from build123d import *

# Parameters (mm, degrees)
SKETCH1_R           = 40
BOSS_EXTRUDE1_DEPTH = 100
SKETCH2_R           = 30
SKETCH2_R_2         = 15
BOSS_EXTRUDE2_DEPTH = 50
SKETCH1_3_R         = 15
CUT_EXTRUDE1_DEPTH  = 15
BOSS_EXTRUDE3_START = 50
SKETCH2_4_R         = 15
BOSS_EXTRUDE3_DEPTH = 15


with BuildPart() as part:
    # Sketch1 → Boss-Extrude1 (new body)
    with BuildSketch(Plane(origin=(0, 0, 0), x_dir=(1, 0, 0), z_dir=(0, 1, 0))):
        with Locations(Location((0, 0, 0), (0, 0, 270))):
            Circle(SKETCH1_R)
    extrude(amount=BOSS_EXTRUDE1_DEPTH)

    # Sketch2 → Boss-Extrude2 (add)
    with BuildSketch(Plane.XY):
        with Locations(Location((0, 60, 0), (0, 0, 180))):
            Circle(SKETCH2_R)
        with Locations((0, 60)):
            Circle(SKETCH2_R_2, mode=Mode.SUBTRACT)
        with Locations((0, 60)):
            Circle(SKETCH2_R_2)
    extrude(amount=BOSS_EXTRUDE2_DEPTH)

    # Sketch1<3> → Cut-Extrude1 (cut)
    with BuildSketch(Plane(origin=(0, 0, 0), x_dir=(1, 0, 0), z_dir=(0, 1, 0))):
        with Locations(Location((0, 0, 0), (0, 0, 270))):
            Circle(SKETCH1_3_R)
    extrude(amount=CUT_EXTRUDE1_DEPTH, mode=Mode.SUBTRACT)

    # Sketch2<4> → Boss-Extrude3 (add)
    with BuildSketch(Plane.XY.offset(BOSS_EXTRUDE3_START)):
        with Locations((0, 60)):
            Circle(SKETCH2_4_R)
    extrude(amount=BOSS_EXTRUDE3_DEPTH)


solid = part.part
Could you check a few things on this model? Use its own coordinates, in mm. A direction names the side the tool comes from. Give positions to 0.01 mm unless a question says otherwise; leave off trailing zeros. Order: outer loops, then holes, each group sorted by start corner. A loop starts at its lowest first (then second) coordinate and runs counter-clockwise, first axis right, second up. Notation, with made-up numbers: (36.5, 69) - (80.5, 69) arc R22 cw to (80.5, 89) - close; hole circle Ø1 at (88.25, -26.5). An arc over 180 degrees is marked (long way). Return JSON: item names as keys, results as strings. Group by question number.
Q1. Suppose I cut it at B-B, the plane x = 0. Please give me the cut outline in (y, z), and give its area (3 significant figures).
Q2. Suppose I cut it at D-D, the plane y = 12.5. Please give me the cut outline in (x, z).
Q3. Will these pins go through, and if not, where does the flat tip stop? pin 1 Ø12 at (x, y) = (-21.5, 11) entering from +Z; pin 2 Ø9 at (x, z) = (-6.5, -2.5) entering from -Y; pin 3 Ø5 at (x, y) = (13, 20) entering from +Z.
Q4. Suppose I cut it at A-A, the plane z = 0. Please give me the cut outline in (x, y).
Q5. Which directions (+Z, -Z, +X, -X, +Y, -Y) give clear straight access to the entire face, cutting with the end or side of a thin tool? Please do faces 4 (the face through (-3.252, 45.357, 57.395)), 5 (the face through (0.66, 7.395, -14.985)), 6 (the face through (0, 60, 65)).
Q6. Thinking about a two-plate mould opening in X: for faces 1 (the face through (1, 100, -1)), 2 (the face through (0, 15, 0)), 3 (the face through (1.76, 49.3, -39.96)), which applies, pulls with the +X half, pulls with the -X half, needs draft (parallel to the pull), parting line crosses it, or undercut?
Q7. Please list where these lines run through material, in increasing order: line 1 along X through (y, z) = (10.5, 0); line 2 along Z through (x, y) = (-12.5, 8); line 3 along Y through (x, z) = (-10.5, 1.5). Write a range as [from, to].
Q8. Suppose I cut it at C-C, the plane y = 60. Please give me the cut outline in (x, z).
Resolved:
{
 "1": {"outline": "(0, -40) - (100, -40) - (100, 40) - (90, 40) - (90, 50) - (75, 50) - (75, 65) - (45, 65) - (45, 50) - (30, 50) - (30, 40) - (0, 40) - (0, 15) - (15, 15) - (15, -15) - (0, -15) - close", "area": "8,600 mm2"},
 "2": {"outline": "circle Ø80 at (0, 0); hole circle Ø30 at (0, 0)"},
 "3": {"pin 1": "stops at z = 36.87", "pin 2": "stops at y = 15", "pin 3": "stops at z = 38.6"},
 "4": {"outline": "(-40, 0) - (-15, 0) - (-15, 15) - (15, 15) - (15, 0) - (40, 0) - (40, 100) - (-40, 100) - close"},
 "5": {"face 4": "+Z", "face 5": "-Y", "face 6": "+Z, +X, -X, +Y, -Y"},
 "6": {"face 1": "needs draft", "face 2": "undercut", "face 3": "parting line crosses it"},
 "7": {"line 1": "x = [-40, -15], [15, 40]", "line 2": "z = [-38, -8.29], [8.29, 38]", "line 3": "y = [15, 100]"},
 "8": {"outline": "(-30, 26.46) arc R40 ccw (long way) to (30, 26.46) - (30, 50) - (15, 50) - (15, 65) - (-15, 65) - (-15, 50) - (-30, 50) - close"}
}
